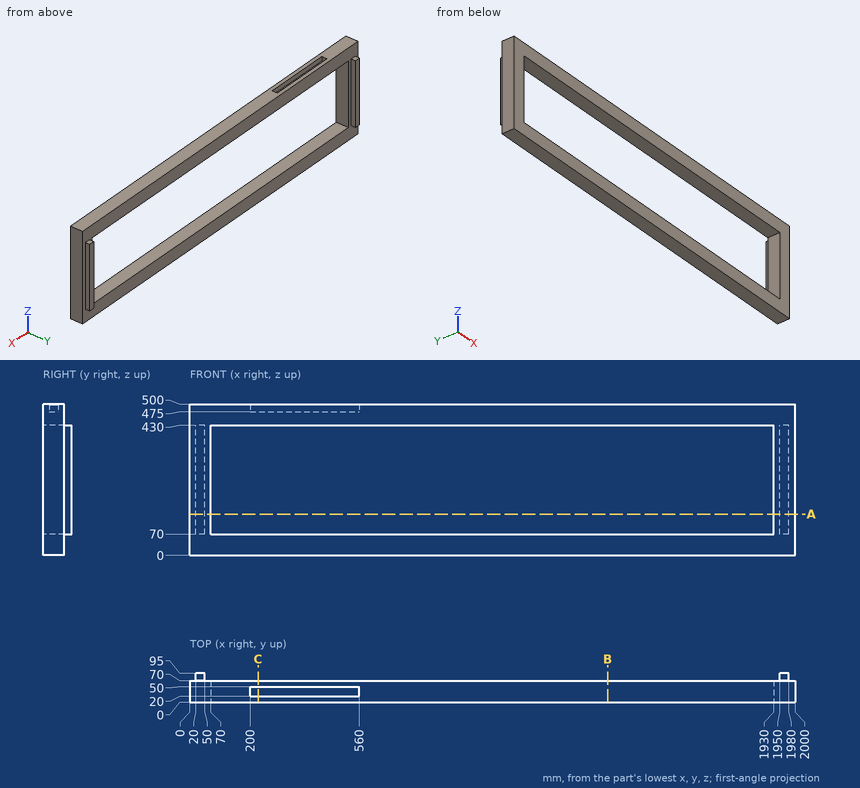
For this review, use the dimensioned drawing (mm, ordinates from the lowest corner) and the shaded views. Round coordinates to 2 decimals unless told otherwise and drop trailing zeros. Write each loop counter-clockwise with the first axis right and the second up, starting at its lowest first coordinate (ties: lowest second). Pieces come first, ordered by that corner, then holes. Notation, with made-up numbers: (-38, 15.5) -> (-10, 15.5) arc R20 ccw to (-10, 46.5) -> close; hole circle Ø7 at (54.25, -27.5). An arc over 180 degrees is marked (long way). Use CSV: the item, a comma, the result in double quotes.
(1) Consider section C-C, the plane x = 226. Give the boundary of the cut face in (y, z).
Computed values:
outline,"(0, 0) -> (70, 0) -> (70, 70) -> (0, 70) -> close; (0, 430) -> (70, 430) -> (70, 500) -> (50, 500) -> (50, 475) -> (20, 475) -> (20, 500) -> (0, 500) -> close"
(2) Consider section B-B, the plane x = 1380.5. Give the boundary of the cut face in (y, z), plus the area to 3 significant figures.
Computed values:
outline,"(0, 0) -> (70, 0) -> (70, 70) -> (0, 70) -> close; (0, 430) -> (70, 430) -> (70, 500) -> (0, 500) -> close"
area,"9,800 mm²"
(3) Consider section A-A, the plane z = 136. Give the boundary of the cut face in (x, y).
Computed values:
outline,"(0, 0) -> (70, 0) -> (70, 70) -> (50, 70) -> (50, 95) -> (20, 95) -> (20, 70) -> (0, 70) -> close; (1930, 0) -> (2000, 0) -> (2000, 70) -> (1980, 70) -> (1980, 95) -> (1950, 95) -> (1950, 70) -> (1930, 70) -> close"
(4) Clearance check with flat-ended pins moving along their axes: P1, Ø7.5, axis at x = 35.5, y = 79.5, coming from the -Z side; P2, Ø1.5, axis at y = 79.5, z = 291, coming from the +X side; P3, Ø7.5, axis at y = 85, z = 334, coming from the -X side. State where each tip first meets the part, or that it passes through.
Computed values:
P1,"z = 70"
P2,"x = 1980"
P3,"x = 20"
(5) To check wall thickness, follow L1, parallel to Z at x = 814.5, y = 22.5; L2, parallel to X at y = 50, z = 345; L3, parallel to Y at x = 813.5, z = 443.5. State the ranges of each line that lie inside material, in increasing order. Write a range as [from, to].
Computed values:
L1,"[0, 70], [430, 500]"
L2,"[0, 70], [1930, 2000]"
L3,"[0, 70]"
